Verification items for the finished model (mm, model axes). A direction names the side the tool comes from. Round coordinates to 2 decimals unless told otherwise and drop trailing zeros. Write each loop counter-clockwise with the first axis right and the second up, starting at its lowest first coordinate (ties: lowest second). Pieces come first, ordered by that corner, then holes. Notation, with made-up numbers: (75, 45.25) - (96, 45.25) arc R35 cw to (96, 84.25) - close; hole circle Ø9 at (-16, 18). An arc over 180 degrees is marked (long way). Answer as a JSON object with one key per item and string values.
```python
from build123d import *

# Parameters (mm, degrees)
BOSS_EXTRUDE1_DEPTH = 15
CUT_EXTRUDE1_DEPTH  = 16
CUT_EXTRUDE3_START  = -4
CUT_EXTRUDE3_DEPTH  = 12
FILLET2_R           = 0.5
BOSS_EXTRUDE2_DEPTH = 8
SKETCH5_W           = 10.5
SKETCH5_H           = 10.5
CUT_EXTRUDE4_DEPTH  = 7
CUT_EXTRUDE5_DEPTH  = 16
FILLET1_R           = 1


with BuildPart() as part:
    # Sketch1 → Boss-Extrude1 (new body)
    with BuildSketch(Plane(origin=(0, 0, 0), x_dir=(1, 0, 0), z_dir=(0, 1, 0))):
        with BuildLine():
            Line((-57.286267839, -105.443271559), (-68, -124))
            Line((-68, -124), (68, -124))
            Line((68, -124), (57.286267839, -105.443271559))
            ThreePointArc((57.286267839, -105.443271559), (0, -120), (-57.286267839, -105.443271559))
        make_face()
    extrude(amount=BOSS_EXTRUDE1_DEPTH)

    # Sketch2 → Cut-Extrude1 (cut, through all)
    with BuildSketch(Plane(origin=(0, 15, 0), x_dir=(1, 0, 0), z_dir=(0, 1, 0))):
        with BuildLine():
            Line((-52.804159001, -115.380031326), (-55.129159001, -119.407049454))
            ThreePointArc((-55.129159001, -119.407049454), (-58.441770605, -120.294661058), (-59.32938221, -116.982049454))
            Line((-59.32938221, -116.982049454), (-57.00438221, -112.955031326))
            ThreePointArc((-57.00438221, -112.955031326), (-53.691770605, -112.067419722), (-52.804159001, -115.380031326))
        make_face()
        with BuildLine():
            Line((52.804159001, -115.380031326), (55.129159001, -119.407049454))
            ThreePointArc((55.129159001, -119.407049454), (58.441770605, -120.294661058), (59.32938221, -116.982049454))
            Line((59.32938221, -116.982049454), (57.00438221, -112.955031326))
            ThreePointArc((57.00438221, -112.955031326), (53.691770605, -112.067419722), (52.804159001, -115.380031326))
        make_face()
    extrude(amount=-CUT_EXTRUDE1_DEPTH, mode=Mode.SUBTRACT)

    # Sketch3 → Cut-Extrude3 (cut, through all)
    with BuildSketch(Plane(origin=(0, 15, 0), x_dir=(1, 0, 0), z_dir=(0, 1, 0)).offset(CUT_EXTRUDE3_START)):
        with BuildLine():
            Line((-51.019656288, -116.439181962), (-53.319656288, -120.422898819))
            ThreePointArc((-53.319656288, -120.422898819), (-59.466770605, -122.070013136), (-61.113884922, -115.922898819))
            Line((-61.113884922, -115.922898819), (-58.813884922, -111.939181962))
            ThreePointArc((-58.813884922, -111.939181962), (-52.666770605, -110.292067644), (-51.019656288, -116.439181962))
        make_face()
        with BuildLine():
            Line((51.019656288, -116.439181962), (53.319656288, -120.422898819))
            ThreePointArc((53.319656288, -120.422898819), (59.466770605, -122.070013136), (61.113884922, -115.922898819))
            Line((61.113884922, -115.922898819), (58.813884922, -111.939181962))
            ThreePointArc((58.813884922, -111.939181962), (52.666770605, -110.292067644), (51.019656288, -116.439181962))
        make_face()
    extrude(amount=-CUT_EXTRUDE3_DEPTH, mode=Mode.SUBTRACT)

    # Fillet2
    fillet2_edges = [part.edges().sort_by_distance(p)[0] for p in [
        (-58.16688221, 11, 114.96854039),
        (53.966659001, 11, 117.39354039),
        (-52.666770605, 11, 110.292067644),
        (-59.963884922, 11, 113.93104039),
        (-59.466770605, 11, 122.070013136),
        (-52.169656288, 11, 118.43104039),
        (-53.691770605, 11, 112.067419722),
        (-53.966659001, 11, 117.39354039),
        (-58.441770605, 11, 120.294661058),
        (52.666770605, 11, 110.292067644),
        (52.169656288, 11, 118.43104039),
        (59.466770605, 11, 122.070013136),
        (59.963884922, 11, 113.93104039),
        (58.16688221, 11, 114.96854039),
        (53.691770605, 11, 112.067419722),
        (58.441770605, 11, 120.294661058),
    ]]
    fillet(fillet2_edges, radius=FILLET2_R)

    # Sketch4 → Boss-Extrude2 (add)
    with BuildSketch(Plane(origin=(0, 15, 0), x_dir=(1, 0, 0), z_dir=(0, 1, 0))):
        with BuildLine():
            Line((-35.015731887, -89.386232276), (-55, -124))
            Line((-55, -124), (55, -124))
            Line((55, -124), (35.015731887, -89.386232276))
            ThreePointArc((35.015731887, -89.386232276), (0, -96), (-35.015731887, -89.386232276))
        make_face()
    extrude(amount=-BOSS_EXTRUDE2_DEPTH)

    # Sketch5 → Cut-Extrude4 (cut)
    with BuildSketch(Plane.XZ.offset(-7)):
        with Locations((0, 108)):
            Rectangle(SKETCH5_W, SKETCH5_H)
        Polygon((17.998277994, 101.297517192), (20.360264064, 111.528402872), (30.591149745, 109.166416802), (28.229163674, 98.935531121), align=None)
        Polygon((-17.998277994, 101.297517192), (-20.360264064, 111.528402872), (-30.591149745, 109.166416802), (-28.229163674, 98.935531121), align=None)
    extrude(amount=-CUT_EXTRUDE4_DEPTH, mode=Mode.SUBTRACT)

    # Sketch6 → Cut-Extrude5 (cut, through all)
    with BuildSketch(Plane.XZ):
        Polygon((63.716770605, 116.581229068), (63.716770605, 124), (68, 124), align=None)
        Polygon((-68, 124), (-63.716770605, 116.581229068), (-63.716770605, 124), align=None)
    extrude(amount=-CUT_EXTRUDE5_DEPTH, mode=Mode.SUBTRACT)

    # Fillet1
    fillet1_edges = [part.edges().sort_by_distance(p)[0] for p in [
        (35.015731887, 11, 89.386232276),
        (-35.015731887, 11, 89.386232276),
        (47.124753912, 11, 110.359673653),
        (-47.124753912, 11, 110.359673653),
        (63.716770605, 7.5, 116.581229068),
        (63.716770605, 7.5, 124),
        (-63.716770605, 7.5, 124),
        (-63.716770605, 7.5, 116.581229068),
        (57.286267839, 7.5, 105.443271559),
        (-57.286267839, 7.5, 105.443271559),
    ]]
    fillet(fillet1_edges, radius=FILLET1_R)


solid = part.part
```
1. Go/stop test with flat-tipped pins: pin 1 (1.5 mm diameter, centred on x = 45, y = 2, fed in from -Z); pin 2 (6.5 mm diameter, centred on x = 25.5, z = 105.5, fed in from -Y); pin 3 (2 mm diameter, centred on y = 9, z = 108, fed in from -X). Record where each tip stops, or that it passes through.
Completed:
{"pin 1": "stops at z = 110.94", "pin 2": "stops at y = 14", "pin 3": "stops at x = -59.34"}
2. Cross-section at A-A (y = 5). Record the boundary of the cut face in (x, z).
Completed:
{"outline": "(-63.72, 116.85) arc R1 ccw to (-63.58, 116.35) - (-57.77, 106.28) arc R1 ccw to (-56.44, 105.9) arc R120 cw to (56.44, 105.9) arc R1 ccw to (57.77, 106.28) - (63.58, 116.35) arc R1 ccw to (63.72, 116.85) - (63.72, 123) arc R1 ccw to (62.72, 124) - (-62.72, 124) arc R1 ccw to (-63.72, 123) - close; hole (-61.11, 115.92) - (-58.81, 111.94) arc R4.5 ccw to (-51.02, 116.44) - (-53.32, 120.42) arc R4.5 ccw to start; hole (51.02, 116.44) arc R4.5 ccw to (58.81, 111.94) - (61.11, 115.92) arc R4.5 ccw to (53.32, 120.42) - close"}
3. Cross-section at D-D (x = -41). Record the boundary of the cut face in (y, z).
Completed:
{"outline": "(0, 112.78) - (7, 112.78) - (7, 99.75) - (15, 99.75) - (15, 124) - (0, 124) - close"}
4. Cross-section at C-C (x = 26). Record the boundary of the cut face in (y, z), plus the area to 3 significant figures.
Completed:
{"outline": "(0, 117.15) - (7, 117.15) - (7, 110.23) - (14, 110.23) - (14, 99.45) - (7, 99.45) - (7, 92.41) - (15, 92.41) - (15, 124) - (0, 124) - close", "area": "225 mm^2"}
5. Cross-section at B-B (z = 94.5). Record the boundary of the cut face in (x, y), plus the area to 3 significant figures.
Completed:
{"outline": "(-37.97, 7) - (-16.9, 7) - (-16.9, 15) - (-37.97, 15) - close; (16.9, 7) - (37.97, 7) - (37.97, 15) - (16.9, 15) - close", "area": "337 mm^2"}
6. Mould release check, pull along X, two halves, no side actions. Record for faces 1 (the face through (0, 10, 102.75)), 2 (the face through (-63.717, 7, 120)), 3 (the face through (-1, 8, 124)): released by +X, released by -X, zero draft, split by the parting line, or undercut.
Completed:
{"face 1": "undercut", "face 2": "released by -X", "face 3": "zero draft"}
7. Access from +Z, -Z, +X, -X, +Y, -Y to the whole of each face (thin tool, end or side, straight path). Record for faces 4 (the face through (-1, 15, 110)), 5 (the face through (24, 14, 105)), 6 (the face through (0, 11, 96)), 7 (the face through (-1, 7, 101)), 8 (the face through (53.95, 13.274, 117.365)).
Completed:
{"face 4": "+Z, -Z, +X, -X, +Y", "face 5": "-Y", "face 6": "-Z, +Y, -Y", "face 7": "-Z, -Y", "face 8": "+Y, -Y"}
8. Material ranges on probe 1 along Y at (x, z) = (42, 104.5); probe 2 along X at (y, z) = (9.25, 112.5); probe 3 along Y at (x, z) = (4.5, 112.5), recorded low to high. Write a range as from..to.
Completed:
{"probe 1": "y = 7..15", "probe 2": "x = -61.36..-59.14, -50.75..-5.25, 5.25..50.75, 59.14..61.36", "probe 3": "y = 14..15"}
